```python
from build123d import *

# Parameters (mm, degrees)
SKETCH_1_R        = 10
EXTRUDE_1_DEPTH   = 5
SKETCH_2_R        = 7.5
EXTRUDE_2_DEPTH   = 10
OTHER_START       = 5
OTHER_1_OUTLINE_R = 1.8
OTHER_1_DEPTH     = 10


# Read off the part's stored shape, not the designer's step: 高级异型孔1
with BuildPart() as part:
    # 草图1 → 凸台-拉伸1 (new body)
    with BuildSketch(Plane(origin=(0, 0, 0), x_dir=(1, 0, 0), z_dir=(0, 1, 0))):
        with Locations(Location((0, 0, 0), (0, 0, 270))):
            Circle(SKETCH_1_R)
    extrude(amount=EXTRUDE_1_DEPTH)

    # 草图2 → 凸台-拉伸2 (add)
    with BuildSketch(Plane(origin=(0, 5, 0), x_dir=(1, 0, 0), z_dir=(0, 1, 0))):
        with Locations(Location((0, 0, 0), (0, 0, 270))):
            Circle(SKETCH_2_R)
    extrude(amount=EXTRUDE_2_DEPTH)

    # 高级异型孔1 outline → 高级异型孔1 (cut)
    with BuildSketch(Plane(origin=(0, 0, 0), x_dir=(1, 0, 0), z_dir=(0, 1, 0)).offset(OTHER_START)):
        Circle(OTHER_1_OUTLINE_R)
    extrude(amount=OTHER_1_DEPTH, mode=Mode.SUBTRACT)


solid = part.part
```
Here's how the part is built. I have some questions about the finished solid (model axes, mm). A direction names the side the tool comes from. Coordinates: 2 decimals unless noted, no trailing zeros. Order: outer loops, then holes, each group sorted by start corner. A loop starts at its lowest first (then second) coordinate and runs counter-clockwise, first axis right, second up.
1) Imagine slicing it at C-C on y = 10. List the corners of the cut face in (x, z) for me.
2) Imagine slicing it at D-D on x = -6. List the corners of the cut face in (y, z) for me, and give its area (3 significant figures).
3) I need wall thicknesses on line 1 (X direction, y = 8, z = 0); line 2 (Y direction, x = 8.5, z = -1); line 3 (Z direction, x = -1.75, y = 3.75). Which ranges of each line are inside material? Lowest first, please.
4) Which directions (+Z, -Z, +X, -X, +Y, -Y) give clear straight access to the entire face, cutting with the end or side of a thin tool? Please do faces 1 (the face through (7, 5, 4)), 2 (the face through (-2, 15, 2)).
5) Imagine slicing it at B-B on x = 0. List the corners of the cut face in (y, z) for me, and give its area (3 significant figures).
6) Imagine slicing it at A-A on z = 0. List the corners of the cut face in (x, y) for me.
7) We'd pull the mould along Z, two halves only. Please class faces 3 (the face through (1.717, 9.93, -0.541)), 4 (the face through (0, 0, 0)), 5 (the face through (-9.76, 2.46, -2.17)), 6 (the face through (0, 5, 0)): +Z half, -Z half, draft (parallel to the pull), parting line (faces both ways), or undercut.
8) Will these pins go through, and if not, where does the flat tip stop? pin 1 (5 mm diameter, centred on y = 6, z = -1.5, fed in from +X); pin 2 (2 mm diameter, centred on y = 4.5, z = 5, fed in from +X); pin 3 (5 mm diameter, centred on y = 11, z = 5.5, fed in from -X); pin 4 (4 mm diameter, centred on y = 8.5, z = 7, fed in from +X).
Response values:
1. outline: circle Ø15 at (0, 0); hole circle Ø3.6 at (0, 0)
2. outline: (0, -8) - (5, -8) - (5, -4.5) - (15, -4.5) - (15, 4.5) - (5, 4.5) - (5, 8) - (0, 8) - close
2. area: 170 mm2
3. line 1: x = -7.5 to -1.8, 1.8 to 7.5
3. line 2: y = 0 to 5
3. line 3: z = -9.85 to 9.85
4. face 1: +Y
4. face 2: +Z, -Z, +X, -X, +Y
5. outline: (0, -10) - (5, -10) - (5, -7.5) - (15, -7.5) - (15, -1.8) - (5, -1.8) - (5, 1.8) - (15, 1.8) - (15, 7.5) - (5, 7.5) - (5, 10) - (0, 10) - close
5. area: 214 mm2
6. outline: (-10, 0) - (10, 0) - (10, 5) - (7.5, 5) - (7.5, 15) - (1.8, 15) - (1.8, 5) - (-1.8, 5) - (-1.8, 15) - (-7.5, 15) - (-7.5, 5) - (-10, 5) - close
7. face 3: undercut
7. face 4: draft
7. face 5: parting line
7. face 6: undercut
8. pin 1: stops at x = 10
8. pin 2: stops at x = 9.17
8. pin 3: stops at x = -6.87
8. pin 4: stops at x = 5.59
